Could you check a few things on this drawing? It's one solid part, dimensions in mm from its lowest x, y, z. Coordinates: 2 decimals unless noted, no trailing zeros. Order: outer loops, then holes, each group sorted by start corner. A loop starts at its lowest first (then second) coordinate and runs counter-clockwise, first axis right, second up. Notation, with made-up numbers: (12, 51.5) - (61, 51.5) arc R28 ccw to (61, 85.5) - close; hole circle Ø10 at (-6.75, 22.5). An arc over 180 degrees is marked (long way). Return JSON: item names as keys, results as strings. Group by question number.
1) Imagine slicing it at D-D (y = 139). Write out the boundary of the cut face in (x, z), and give its area (3 significant figures).
2) For pin 1 Ø1 at (x, z) = (63, 2.5) entering from -Y; pin 2 Ø1.6 at (x, z) = (80.5, 1.5) entering from +Y; pin 3 Ø1.6 at (x, z) = (93, 2) entering from +Y, each with a flat end and sliding along its axis, tell me the tip position at first contact or that it passes through.
3) Imagine slicing it at A-A (x = 75). Write out the boundary of the cut face in (y, z).
4) If I drill on line 1 along Y through (x, z) = (75, 0.75); line 2 along Y through (x, z) = (85, 1.3); line 3 along Y through (x, z) = (101.5, 2.4), over which ranges is the centre line in solid material (lowest first)?
5) Imagine slicing it at C-C (z = 0.9). Write out the boundary of the cut face in (x, y).
6) Imagine slicing it at B-B (y = 75). Write out the boundary of the cut face in (x, z), and give its area (3 significant figures).
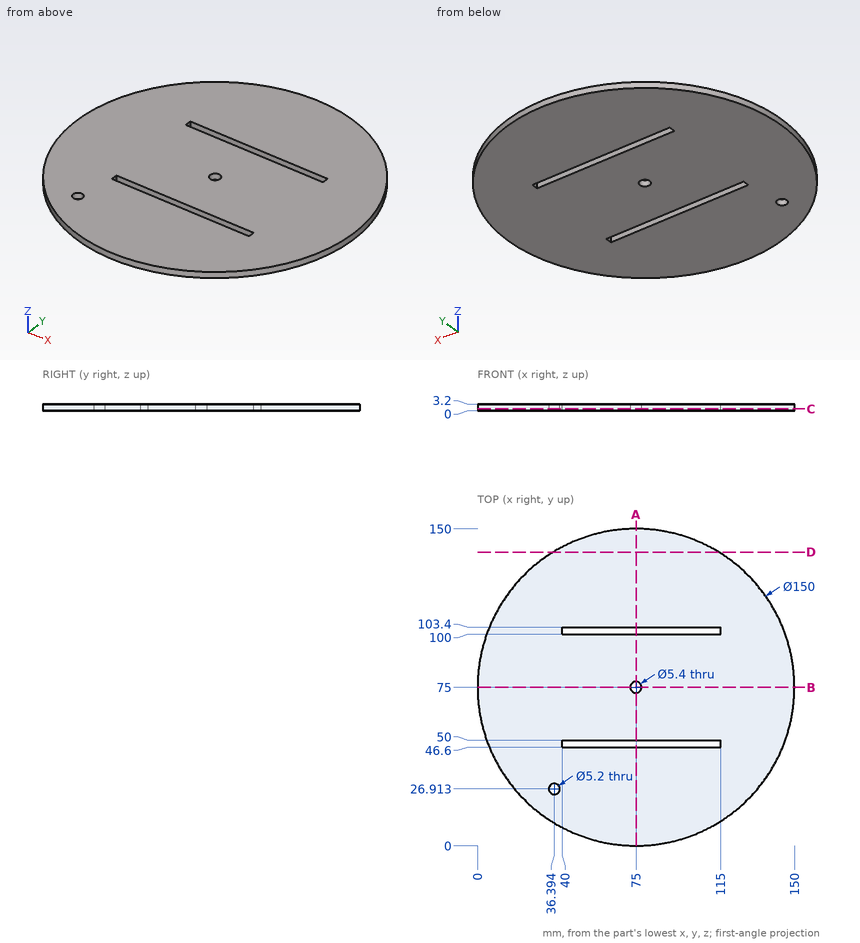
Calculated:
{
 "1": {"outline": "(35.9, 0) - (114.1, 0) - (114.1, 3.2) - (35.9, 3.2) - close", "area": "250 mm2"},
 "2": {"pin 1": "y = 0.89", "pin 2": "y = 149.85", "pin 3": "y = 148"},
 "3": {"outline": "(0, 0) - (46.6, 0) - (46.6, 3.2) - (0, 3.2) - close; (50, 0) - (72.3, 0) - (72.3, 3.2) - (50, 3.2) - close; (77.7, 0) - (100, 0) - (100, 3.2) - (77.7, 3.2) - close; (103.4, 0) - (150, 0) - (150, 3.2) - (103.4, 3.2) - close"},
 "4": {"line 1": "0 to 46.6, 50 to 72.3, 77.7 to 100, 103.4 to 150", "line 2": "0.67 to 46.6, 50 to 100, 103.4 to 149.33", "line 3": "4.84 to 46.6, 50 to 100, 103.4 to 145.16"},
 "5": {"outline": "circle Ø150 at (75, 75); hole circle Ø5.2 at (36.39, 26.91); hole (40, 46.6) - (115, 46.6) - (115, 50) - (40, 50) - close; hole (40, 100) - (115, 100) - (115, 103.4) - (40, 103.4) - close; hole circle Ø5.4 at (75, 75)"},
 "6": {"outline": "(0, 0) - (72.3, 0) - (72.3, 3.2) - (0, 3.2) - close; (77.7, 0) - (150, 0) - (150, 3.2) - (77.7, 3.2) - close", "area": "463 mm2"}
}
